Job drawing, mm, ordinate dimensions from the low corner. One solid piece. A direction names the side the tool comes from. Round coordinates to 2 decimals unless told otherwise and drop trailing zeros. Loops run counter-clockwise (first coordinate to the right, second up) from the corner with the lowest first, then second, coordinate; pieces in that order, holes last.
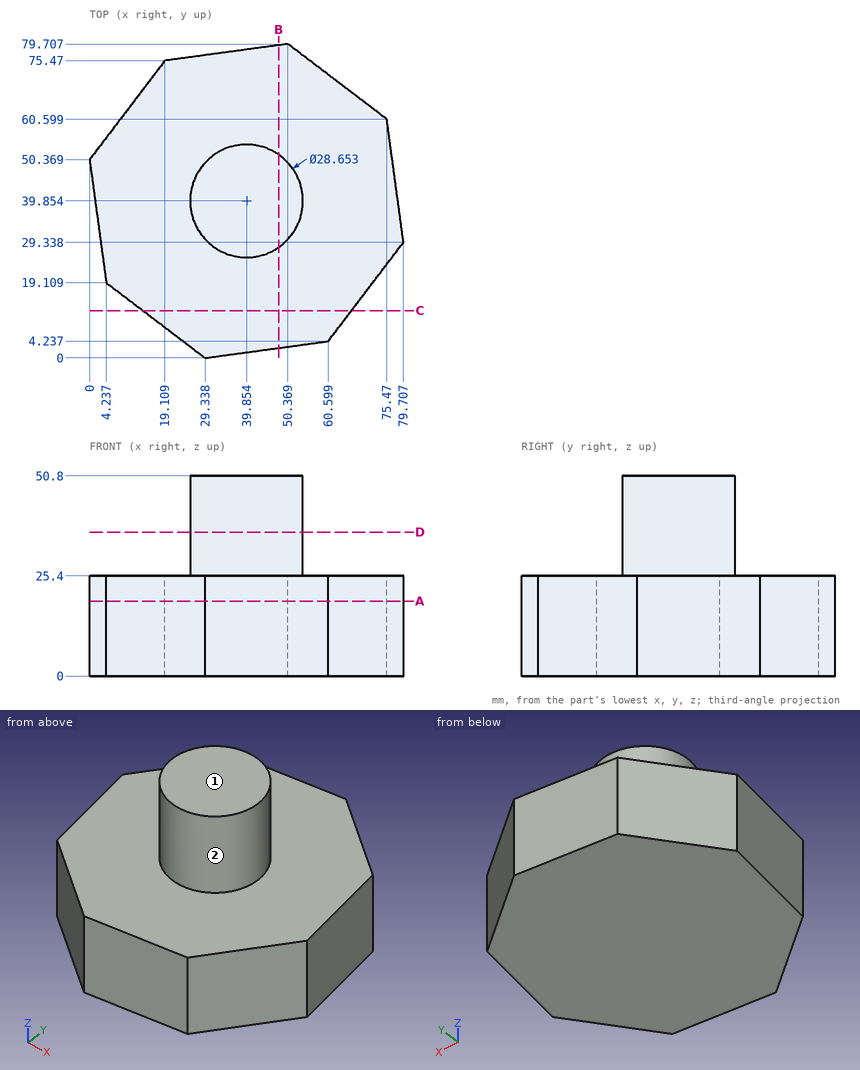
(1) Slice it at C-C on y = 12. List the corners of the cut face in (x, z) (1 decimal).
Responses:
outline: (13.6, 0) - (66.5, 0) - (66.5, 25.4) - (13.6, 25.4) - close
(2) Which spindle directions (+Z, -Z, +X, -X, +Y, -Y) get a long thin tool onto all of the face, cutting with end or side? Do the marked faces 1 and 2. Say none if no direction does.
Responses:
face 1: +Z, +X, -X, +Y, -Y
face 2: +Z
(3) Slice it at B-B on x = 48. List the corners of the cut face in (y, z).
Responses:
outline: (2.53, 0) - (79.39, 0) - (79.39, 25.4) - (51.64, 25.4) - (51.64, 50.8) - (28.07, 50.8) - (28.07, 25.4) - (2.53, 25.4) - close
(4) Pin check, flat tips, straight feed: P1, Ø12, axis at y = 57.5, z = 26.5, coming from the -X side; P2, Ø8, axis at x = 70.5, z = 19.5, coming from the -Y side; P3, Ø8, axis at x = 24, z = 41, coming from the +Y side; P4, Ø6, axis at x = 27, y = 51.5, coming from the -Z side. Stop position of each tip, or through.
Responses:
P1: stops at x = 0.94
P2: stops at y = 11.99
P3: stops at y = 47.9
P4: stops at z = 0
(5) Probe line 1 (Z direction, x = 41, y = 25); line 2 (X direction, y = 28.5, z = 11) (1 decimal); line 3 (Y direction, x = 4.5, z = 10) (1 decimal). List the from-to ranges inside material, lowest first.
Responses:
line 1: z = 0 to 25.4
line 2: x = 3 to 79.1
line 3: y = 18.9 to 56.3
(6) Slice it at A-A on z = 19. List the corners of the cut face in (x, y), plus the area to 4 significant figures.
Responses:
outline: (0, 50.37) - (4.24, 19.11) - (29.34, 0) - (60.6, 4.24) - (79.71, 29.34) - (75.47, 60.6) - (50.37, 79.71) - (19.11, 75.47) - close
area: 4,805 mm2
(7) Slice it at D-D on z = 36.5. List the corners of the cut face in (x, y), plus the area to 3 significant figures.
Responses:
outline: circle Ø28.65 at (39.85, 39.85)
area: 645 mm2
